Source: CAD feature listing. Evaluate the final solid. Frame: model axes, mm. Face numbers are marked on the shaded views. Coordinates: 2 decimals unless noted, no trailing zeros. Order: outer loops, then holes, each group sorted by start corner. A loop starts at its lowest first (then second) coordinate and runs counter-clockwise, first axis right, second up. Notation, with made-up numbers: (43.5, 83) - (98.5, 83) arc R26 cw to (98.5, 118) - close; hole circle Ø2 at (-11.75, 17.5). An arc over 180 degrees is marked (long way). One line per question, with ' | ' between items. Start each with the question number.
(1) Contact query for flat-ended pins moving along their axis: P1, Ø6, axis at x = -7.5, y = -2, coming from the +Z side; P2, Ø1.5, axis at x = -7.5, y = -4, coming from the +Z side; P3, Ø6, axis at x = 3, z = 0.5, coming from the +Y side; P4, Ø2, axis at x = -4, y = -4.5, coming from the +Z side. Output: stop coordinate, or through.
(2) Section B-B (z = 0). Return the cut outline in (x, y).
(3) Section D-D (y = -1). Return the cut outline in (x, z), then the cut area to 3 significant figures.
(4) Draft query along Z for the marked faces 1, 2 and 3. Return one class per face: +Z half, -Z half, draft (parallel to the pull), parting line (faces both ways), or undercut.
(5) Section C-C (y = -5). Return the cut outline in (x, z), then the cut area to 3 significant figures.
(6) Section A-A (x = 0). Return the cut outline in (y, z), then the cut area to 4 significant figures.
(7) Line query: line 1 along Z through (x, y) = (-0.25, -8); line 2 along X through (y, z) = (-6.5, 1.75); line 3 along Z through (x, y) = (-9, -7.25). Output: solid intervals per line, ascending.
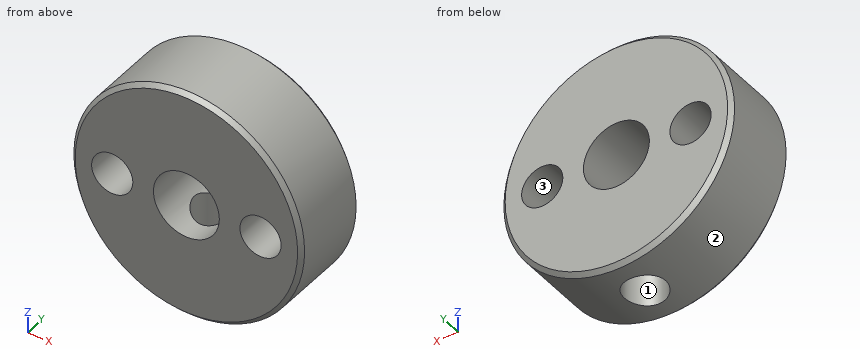
from build123d import *

# Parameters (mm, degrees)
F0_R     = 2.5
F0_R_2   = 14
F1_DEPTH = 10
F2_SIZE  = 0.5
F3_R     = 2.5
F4_DEPTH = 25


with BuildPart() as f1:
    # F0 (on Front) → F1 (new body)
    with BuildSketch(Plane.XZ):
        with Locations((-9, 0)):
            Circle(F0_R)
        with BuildLine():
            ThreePointArc((11.5, 0), (9, 2.5), (6.5, 0))
            ThreePointArc((6.5, 0), (9, -2.5), (11.5, 0))
        make_face()
        Circle(F0_R_2)
        with Locations((-9, 0)):
            Circle(F0_R, mode=Mode.SUBTRACT)
        with BuildLine():
            ThreePointArc((-4, 0), (0, 4), (4, 0))
            ThreePointArc((4, 0), (0, -4), (-4, 0))
        make_face(mode=Mode.SUBTRACT)
        with BuildLine():
            ThreePointArc((11.5, 0), (9, -2.5), (6.5, 0))
            ThreePointArc((6.5, 0), (9, 2.5), (11.5, 0))
        make_face(mode=Mode.SUBTRACT)
    extrude(amount=F1_DEPTH)

    # F2
    f2_edges = [f1.edges().sort_by_distance(p)[0] for p in [
        (-14, -10, 0),
        (-14, 0, 0),
    ]]
    chamfer(f2_edges, length=F2_SIZE)

    # F3 (on Top) → F4 (cut)
    with BuildSketch(Plane.XY):
        with Locations((0, -5)):
            Circle(F3_R)
    extrude(amount=-F4_DEPTH, mode=Mode.SUBTRACT)


solid = f1.part
Response values:
1) P1: stops at z = 13.26 | P2: stops at z = 12.27 | P3: stops at y = 0 | P4: stops at z = 13.67
2) outline: (-14, -9.5) - (-13.5, -10) - (-11.5, -10) - (-11.5, 0) - (-13.5, 0) - (-14, -0.5) - close; (-6.5, -10) - (-4, -10) - (-4, 0) - (-6.5, 0) - close; (4, -10) - (6.5, -10) - (6.5, 0) - (4, 0) - close; (11.5, -10) - (13.5, -10) - (14, -9.5) - (14, -0.5) - (13.5, 0) - (11.5, 0) - close
3) outline: circle Ø28 at (0, 0); hole circle Ø5 at (-9, 0); hole circle Ø8 at (0, 0); hole circle Ø5 at (9, 0) | area: 526 mm²
4) face 1: draft | face 2: parting line | face 3: undercut
5) outline: (-2.5, -13.77) - (-2.5, -3.12) arc R4 cw (long way) to (2.5, -3.12) - (2.5, -13.77) arc R14 ccw (long way) to start; hole circle Ø5 at (-9, 0); hole circle Ø5 at (9, 0) | area: 475 mm²
6) outline: (-10, -13.5) - (-9.5, -14) - (-7.5, -14) - (-7.5, -4) - (-10, -4) - close; (-10, 4) - (0, 4) - (0, 13.5) - (-0.5, 14) - (-9.5, 14) - (-10, 13.5) - close; (-2.5, -14) - (-0.5, -14) - (0, -13.5) - (0, -4) - (-2.5, -4) - close | area: 149.5 mm²
7) line 1: z = -14 to -3.99, 3.99 to 14 | line 2: x = -13.89 to -10.79, -7.21 to -3.6, 3.6 to 7.21, 10.79 to 13.89 | line 3: z = -10.72 to -2.5, 2.5 to 10.72
